Could you check a few things on this model? Use its own coordinates, in mm. Round coordinates to 2 decimals unless told otherwise and drop trailing zeros. Write each loop counter-clockwise with the first axis right and the second up, starting at its lowest first coordinate (ties: lowest second). Pieces come first, ordered by that corner, then holes. Notation, with made-up numbers: (-24, 3.25) - (-6, 3.25) arc R13 cw to (-6, 7.25) - close; hole circle Ø10 at (28.5, 54). An arc over 180 degrees is marked (long way). Write each question's results on one line, items separated by ' | '. Start each with the question number.
(1) Imagine slicing it at A-A on x = -15. Write out the boundary of the cut face in (y, z), then the cut area to 3 significant figures.
(2) Imagine slicing it at D-D on y = 46. Write out the boundary of the cut face in (x, z).
(3) Imagine slicing it at B-B on z = 4.1. State how many separate pieces and enclosed holes the cut face has, then the cut area to 3 significant figures.
(4) Please list where these lines run through material, in increasing order: line 1 (Y direction, x = 0, z = 2.05); line 2 (Y direction, x = 50, z = 4); line 3 (Y direction, x = -0.5, z = 4.75). Write a range as [from, to].
(5) For P1, Ø1.4, axis at x = 35.36, y = -35.36, coming from the -Z side; P2, Ø4, axis at x = -22, y = -9.5, coming from the -Z side; P3, Ø3, axis at x = -15, z = 4.5, coming from the -Y side; P4, Ø2, axis at x = 27.5, z = 1, coming from the -Y side, each with a flat end and sliding along its axis, tell me the tip position at first contact or that it passes through.
```python
from build123d import *

# Parameters (mm, degrees)
SKETCH1_R           = 60.5
SKETCH1_R_2         = 1.25
SKETCH1_R_3         = 8
SKETCH1_R_4         = 1.75
SKETCH1_R_5         = 1.5
BOSS_EXTRUDE1_DEPTH = 6
MOVE_FACE1_BY       = 0.08
MOVE_FACE1_2_BY     = 0.08
MOVE_FACE1_3_BY     = 0.08
MOVE_FACE1_4_BY     = 0.08
MOVE_FACE1_5_BY     = 0.08
MOVE_FACE1_6_BY     = 0.08
MOVE_FACE1_7_BY     = 0.08
MOVE_FACE1_8_BY     = 0.08
MOVE_FACE1_9_BY     = 0.08
MOVE_FACE1_10_BY    = 0.08
MOVE_FACE1_11_BY    = 0.08
MOVE_FACE1_12_BY    = 0.08
MOVE_FACE1_13_BY    = 0.08
MOVE_FACE1_14_BY    = 0.08
MOVE_FACE1_15_BY    = 0.08


with BuildPart() as part:
    # Sketch1 → Boss-Extrude1 (new body)
    with BuildSketch(Plane.XY):
        Circle(SKETCH1_R)
        with Locations((35.355339059, -35.355339059)):
            Circle(SKETCH1_R_2, mode=Mode.SUBTRACT)
        Circle(SKETCH1_R_3, mode=Mode.SUBTRACT)
        with Locations((0, -15)):
            Circle(SKETCH1_R_4, mode=Mode.SUBTRACT)
        with Locations((10.606601718, -10.606601718)):
            Circle(SKETCH1_R_5, mode=Mode.SUBTRACT)
        with Locations((0, -50)):
            Circle(SKETCH1_R_2, mode=Mode.SUBTRACT)
        with Locations((-15, 0)):
            Circle(SKETCH1_R_4, mode=Mode.SUBTRACT)
        with Locations((-10.606601718, -10.606601718)):
            Circle(SKETCH1_R_5, mode=Mode.SUBTRACT)
        with Locations((0, 15)):
            Circle(SKETCH1_R_4, mode=Mode.SUBTRACT)
        with Locations((-10.606601718, 10.606601718)):
            Circle(SKETCH1_R_5, mode=Mode.SUBTRACT)
        with Locations((10.606601718, 10.606601718)):
            Circle(SKETCH1_R_5, mode=Mode.SUBTRACT)
        with Locations((-35.355339059, -35.355339059)):
            Circle(SKETCH1_R_2, mode=Mode.SUBTRACT)
        with Locations((-50, 0)):
            Circle(SKETCH1_R_2, mode=Mode.SUBTRACT)
        with Locations((-35.355339059, 35.355339059)):
            Circle(SKETCH1_R_2, mode=Mode.SUBTRACT)
        with Locations((0, 50)):
            Circle(SKETCH1_R_2, mode=Mode.SUBTRACT)
        with Locations((50, 0)):
            Circle(SKETCH1_R_2, mode=Mode.SUBTRACT)
    extrude(amount=BOSS_EXTRUDE1_DEPTH)

    # Move Face1: a curved face moved outward by 0.08
    add(Solid.thicken(part.faces().sort_by_distance((34.105339059, -35.355339059, 3))[0], MOVE_FACE1_BY))

    # Move Face1 2: a curved face moved outward by 0.08
    add(Solid.thicken(part.faces().sort_by_distance((-8, 0, 3))[0], MOVE_FACE1_2_BY))

    # Move Face1 3: a curved face moved outward by 0.08
    add(Solid.thicken(part.faces().sort_by_distance((-1.75, -15, 3))[0], MOVE_FACE1_3_BY))

    # Move Face1 4: a curved face moved outward by 0.08
    add(Solid.thicken(part.faces().sort_by_distance((9.106601718, -10.606601718, 3))[0], MOVE_FACE1_4_BY))

    # Move Face1 5: a curved face moved outward by 0.08
    add(Solid.thicken(part.faces().sort_by_distance((-1.25, -50, 3))[0], MOVE_FACE1_5_BY))

    # Move Face1 6: a curved face moved outward by 0.08
    add(Solid.thicken(part.faces().sort_by_distance((-36.605339059, -35.355339059, 3))[0], MOVE_FACE1_6_BY))

    # Move Face1 7: a curved face moved outward by 0.08
    add(Solid.thicken(part.faces().sort_by_distance((-16.75, 0, 3))[0], MOVE_FACE1_7_BY))

    # Move Face1 8: a curved face moved outward by 0.08
    add(Solid.thicken(part.faces().sort_by_distance((-12.106601718, -10.606601718, 3))[0], MOVE_FACE1_8_BY))

    # Move Face1 9: a curved face moved outward by 0.08
    add(Solid.thicken(part.faces().sort_by_distance((-1.75, 15, 3))[0], MOVE_FACE1_9_BY))

    # Move Face1 10: a curved face moved outward by 0.08
    add(Solid.thicken(part.faces().sort_by_distance((-12.106601718, 10.606601718, 3))[0], MOVE_FACE1_10_BY))

    # Move Face1 11: a curved face moved outward by 0.08
    add(Solid.thicken(part.faces().sort_by_distance((9.106601718, 10.606601718, 3))[0], MOVE_FACE1_11_BY))

    # Move Face1 12: a curved face moved outward by 0.08
    add(Solid.thicken(part.faces().sort_by_distance((-51.25, 0, 3))[0], MOVE_FACE1_12_BY))

    # Move Face1 13: a curved face moved outward by 0.08
    add(Solid.thicken(part.faces().sort_by_distance((-36.605339059, 35.355339059, 3))[0], MOVE_FACE1_13_BY))

    # Move Face1 14: a curved face moved outward by 0.08
    add(Solid.thicken(part.faces().sort_by_distance((-1.25, 50, 3))[0], MOVE_FACE1_14_BY))

    # Move Face1 15: a curved face moved outward by 0.08
    add(Solid.thicken(part.faces().sort_by_distance((48.75, 0, 3))[0], MOVE_FACE1_15_BY))


solid = part.part
```
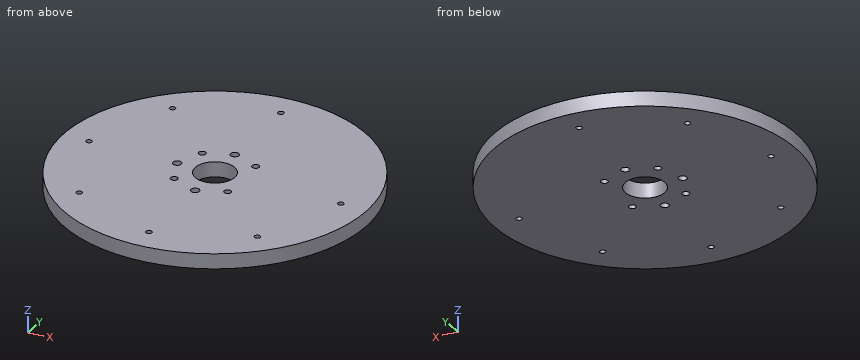
Response:
1) outline: (-58.61, 0) - (-1.67, 0) - (-1.67, 6) - (-58.61, 6) - close; (1.67, 0) - (58.61, 0) - (58.61, 6) - (1.67, 6) - close | area: 683 mm²
2) outline: (-39.3, 0) - (39.3, 0) - (39.3, 6) - (-39.3, 6) - close
3) separate pieces: 1 | enclosed holes: 15 | area: 11,200 mm²
4) line 1: [-60.5, -51.17], [-48.83, -16.67], [-13.33, -7.92], [7.92, 13.33], [16.67, 48.83], [51.17, 60.5] | line 2: [-34.06, -1.17], [1.17, 34.06] | line 3: [-60.5, -51.06], [-48.94, -16.59], [-13.41, -7.9], [7.9, 13.41], [16.59, 48.94], [51.06, 60.5]
5) P1: through | P2: z = 0 | P3: y = -58.97 | P4: y = -54.39
